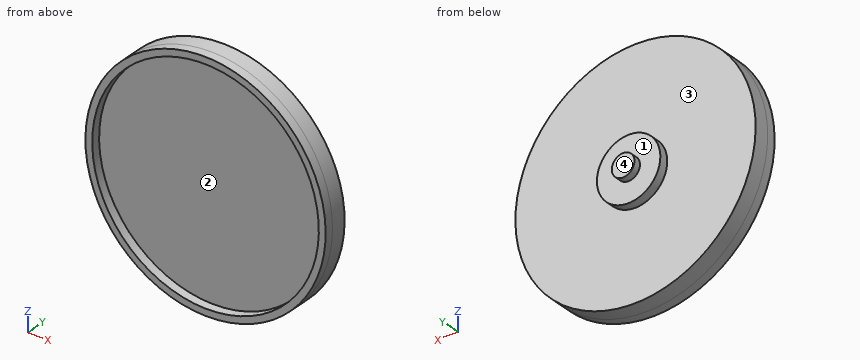
from build123d import *

# Parameters (mm, degrees)
SKETCH1_R           = 26.5
BOSS_EXTRUDE1_DEPTH = 3.5
SKETCH2_R           = 7
BOSS_EXTRUDE2_DEPTH = 2
SKETCH5_R           = 2.5
BOSS_EXTRUDE3_DEPTH = 1.6
BOSS_EXTRUDE4_START = 2
SKETCH6_R           = 26.5
SKETCH6_R_2         = 25
BOSS_EXTRUDE4_DEPTH = 2


with BuildPart() as part:
    # Sketch1 → Boss-Extrude1 (new body)
    with BuildSketch(Plane(origin=(0, 0, 0), x_dir=(1, 0, 0), z_dir=(0, 1, 0))):
        with Locations(Location((0, 0, 0), (0, 0, 270))):
            Circle(SKETCH1_R)
    extrude(amount=BOSS_EXTRUDE1_DEPTH)

    # Sketch2 → Boss-Extrude2 (add)
    with BuildSketch(Plane(origin=(0, 3.5, 0), x_dir=(1, 0, 0), z_dir=(0, 1, 0))):
        with Locations(Location((0, 0, 0), (0, 0, 270))):
            Circle(SKETCH2_R)
    extrude(amount=BOSS_EXTRUDE2_DEPTH)

    # Sketch5 → Boss-Extrude3 (add)
    with BuildSketch(Plane(origin=(0, 5.5, 0), x_dir=(1, 0, 0), z_dir=(0, 1, 0))):
        with Locations(Location((0, 0, 0), (0, 0, 270))):
            Circle(SKETCH5_R)
    extrude(amount=BOSS_EXTRUDE3_DEPTH)

    # Sketch6 → Boss-Extrude4 (add)
    with BuildSketch(Plane.XZ.offset(BOSS_EXTRUDE4_START)):
        with Locations(Location((0, 0, 0), (0, 0, 270))):
            Circle(SKETCH6_R)
        with Locations(Location((0, 0, 0), (0, 0, 270))):
            Circle(SKETCH6_R_2, mode=Mode.SUBTRACT)
    extrude(amount=-BOSS_EXTRUDE4_DEPTH)


solid = part.part
Work out the finished part from the listing and answer in its coordinate system (mm). Face numbers are marked on the shaded views. A direction names the side the tool comes from. Coordinates: 2 decimals unless noted, no trailing zeros. Loops run counter-clockwise (first coordinate to the right, second up) from the corner with the lowest first, then second, coordinate; pieces in that order, holes last. Notation, with made-up numbers: M 44,15 L 81,15 A18 cw 81,20 Z; hole C -20,3.25 d8. An arc over 180 degrees is marked long. Answer in a Markdown table with one row per item. Add a question column.
1. Flat-ended cylindrical pins translate along their axes: P1, Ø1, axis at x = -15.5, y = 3, coming from the +Z side; P2, Ø5, axis at y = -1, z = 8.5, coming from the +X side; P3, Ø4, axis at x = -3, y = 1.5, coming from the +Z side. Find the tip coordinate at first contact, or state that the pin passes through.
2. Find section A-A, the plane z = 0. Write down the section's boundary in (x, y), then the cut area to 4 significant figures.
3. Find section B-B, the plane x = -16. Write down the section's boundary in (y, z).
4. A tool of negligible diameter and unlimited length cuts with its end or side. For the marked faces 3 and 4, from which of +Z, -Z, +X, -X, +Y, -Y can it reach the whole face along a straight path? Write none if from no direction.
5. Consider L1, parallel to X at y = -0.4, z = 0; L2, parallel to Y at x = 8, z = 9; L3, parallel to Y at x = -12, z = -23. Determine where each line is inside the solid, lowest interval first.
6. Find section D-D, the plane z = -13. Write down the section's boundary in (x, y).
7. The mould has two halves that part along Z. Classify the marked faces 1 and 2: pulls with the +Z half, pulls with the -Z half, needs draft (parallel to the pull), parting line crosses it, or undercut.
8. Find section C-C, the plane y = 2.75. Write down the section's boundary in (x, z).
Reported:
| question | item | result |
|---|---|---|
| 1 | P1 | stops at z = 21.85 |
| 1 | P2 | stops at x = 25.81 |
| 1 | P3 | stops at z = 26.48 |
| 2 | outline | M -26.5,-2 L -25,-2 L -25,0 L 25,0 L 25,-2 L 26.5,-2 L 26.5,3.5 L 7,3.5 L 7,5.5 L 2.5,5.5 L 2.5,7.1 L -2.5,7.1 L -2.5,5.5 L -7,5.5 L -7,3.5 L -26.5,3.5 Z |
| 2 | area | 227.5 mm^2 |
| 3 | outline | M -2,-21.12 L 3.5,-21.12 L 3.5,21.12 L -2,21.12 L -2,19.21 L 0,19.21 L 0,-19.21 L -2,-19.21 Z |
| 4 | face 3 | +Y |
| 4 | face 4 | +Z, -Z, +X, -X, +Y |
| 5 | L1 | x = -26.5 to -25, 25 to 26.5 |
| 5 | L2 | y = 0 to 3.5 |
| 5 | L3 | y = -2 to 3.5 |
| 6 | outline | M -23.09,-2 L -21.35,-2 L -21.35,0 L 21.35,0 L 21.35,-2 L 23.09,-2 L 23.09,3.5 L -23.09,3.5 Z |
| 7 | face 1 | needs draft |
| 7 | face 2 | undercut |
| 8 | outline | C 0,0 d53 |
